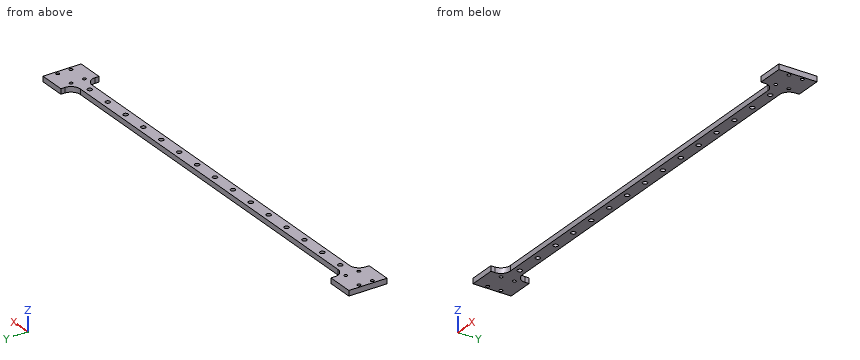
from build123d import *

# Parameters (mm, degrees)
SKETCH1_R           = 1.25
BOSS_EXTRUDE1_DEPTH = 4
FILLET1_R           = 7


with BuildPart() as part:
    # Sketch1 → Boss-Extrude1 (new body)
    with BuildSketch(Plane.XY):
        Polygon((-10, 14.45), (8.795857864, 14.45), (10, 14.45), (10, 4.5), (312, 4.5), (312, 14.45), (312.21, 14.45), (330.795857864, 14.45), (332, 14.45), (332, -14.45), (331.79, -14.45), (313.204142136, -14.45), (312, -14.45), (312, -4.5), (10, -4.5), (10, -14.45), (9.79, -14.45), (-8.795857864, -14.45), (-10, -14.45), (-10, -9.45), (-10, 9.45), align=None)
        with Locations((329.5, -5)):
            Circle(SKETCH1_R, mode=Mode.SUBTRACT)
        with Locations((314.5, 5)):
            Circle(SKETCH1_R, mode=Mode.SUBTRACT)
        with Locations((314.5, -5)):
            Circle(SKETCH1_R, mode=Mode.SUBTRACT)
        with Locations((329.5, 5)):
            Circle(SKETCH1_R, mode=Mode.SUBTRACT)
        with Locations((-7.5, -5)):
            Circle(SKETCH1_R, mode=Mode.SUBTRACT)
        with Locations((-7.5, 5)):
            Circle(SKETCH1_R, mode=Mode.SUBTRACT)
        with Locations((7.5, -5)):
            Circle(SKETCH1_R, mode=Mode.SUBTRACT)
        with Locations((7.5, 5)):
            Circle(SKETCH1_R, mode=Mode.SUBTRACT)
        with BuildLine():
            ThreePointArc((22.05, -1.4), (21, 1.75), (19.95, -1.4))
            ThreePointArc((19.95, -1.4), (21, -1.75), (22.05, -1.4))
        make_face(mode=Mode.SUBTRACT)
        with BuildLine():
            ThreePointArc((42.05, -1.4), (41, 1.75), (39.95, -1.4))
            ThreePointArc((39.95, -1.4), (41, -1.75), (42.05, -1.4))
        make_face(mode=Mode.SUBTRACT)
        with BuildLine():
            ThreePointArc((62.05, -1.4), (61, 1.75), (59.95, -1.4))
            ThreePointArc((59.95, -1.4), (61, -1.75), (62.05, -1.4))
        make_face(mode=Mode.SUBTRACT)
        with BuildLine():
            ThreePointArc((82.05, -1.4), (81, 1.75), (79.95, -1.4))
            ThreePointArc((79.95, -1.4), (81, -1.75), (82.05, -1.4))
        make_face(mode=Mode.SUBTRACT)
        with BuildLine():
            ThreePointArc((102.05, -1.4), (101, 1.75), (99.95, -1.4))
            ThreePointArc((99.95, -1.4), (101, -1.75), (102.05, -1.4))
        make_face(mode=Mode.SUBTRACT)
        with BuildLine():
            ThreePointArc((122.05, -1.4), (121, 1.75), (119.95, -1.4))
            ThreePointArc((119.95, -1.4), (121, -1.75), (122.05, -1.4))
        make_face(mode=Mode.SUBTRACT)
        with BuildLine():
            ThreePointArc((142.05, -1.4), (141, 1.75), (139.95, -1.4))
            ThreePointArc((139.95, -1.4), (141, -1.75), (142.05, -1.4))
        make_face(mode=Mode.SUBTRACT)
        with BuildLine():
            ThreePointArc((162.05, -1.4), (161, 1.75), (159.95, -1.4))
            ThreePointArc((159.95, -1.4), (161, -1.75), (162.05, -1.4))
        make_face(mode=Mode.SUBTRACT)
        with BuildLine():
            ThreePointArc((182.05, -1.4), (181, 1.75), (179.95, -1.4))
            ThreePointArc((179.95, -1.4), (181, -1.75), (182.05, -1.4))
        make_face(mode=Mode.SUBTRACT)
        with BuildLine():
            ThreePointArc((202.05, -1.4), (201, 1.75), (199.95, -1.4))
            ThreePointArc((199.95, -1.4), (201, -1.75), (202.05, -1.4))
        make_face(mode=Mode.SUBTRACT)
        with BuildLine():
            ThreePointArc((222.05, -1.4), (221, 1.75), (219.95, -1.4))
            ThreePointArc((219.95, -1.4), (221, -1.75), (222.05, -1.4))
        make_face(mode=Mode.SUBTRACT)
        with BuildLine():
            ThreePointArc((242.05, -1.4), (241, 1.75), (239.95, -1.4))
            ThreePointArc((239.95, -1.4), (241, -1.75), (242.05, -1.4))
        make_face(mode=Mode.SUBTRACT)
        with BuildLine():
            ThreePointArc((262.05, -1.4), (261, 1.75), (259.95, -1.4))
            ThreePointArc((259.95, -1.4), (261, -1.75), (262.05, -1.4))
        make_face(mode=Mode.SUBTRACT)
        with BuildLine():
            ThreePointArc((282.05, -1.4), (281, 1.75), (279.95, -1.4))
            ThreePointArc((279.95, -1.4), (281, -1.75), (282.05, -1.4))
        make_face(mode=Mode.SUBTRACT)
        with BuildLine():
            ThreePointArc((302.05, -1.4), (301, 1.75), (299.95, -1.4))
            ThreePointArc((299.95, -1.4), (301, -1.75), (302.05, -1.4))
        make_face(mode=Mode.SUBTRACT)
    extrude(amount=BOSS_EXTRUDE1_DEPTH)

    # Fillet1
    fillet1_edges = [part.edges().sort_by_distance(p)[0] for p in [
        (10, 4.5, 2),
        (312, 4.5, 2),
        (312, -4.5, 2),
        (10, -4.5, 2),
    ]]
    fillet(fillet1_edges, radius=FILLET1_R)


solid = part.part
The listing builds one solid part. Answer for the finished solid, in the listing's coordinates (mm). Round coordinates to 2 decimals unless told otherwise and drop trailing zeros. Order: outer loops, then holes, each group sorted by start corner. A loop starts at its lowest first (then second) coordinate and runs counter-clockwise, first axis right, second up. Notation, with made-up numbers: (-10.75, -34.75) -> (7.25, -34.75) arc R11 ccw to (7.25, -19.75) -> close; hole circle Ø4 at (45.5, -23.5). An arc over 180 degrees is marked (long way). One line per item, written item: value.
Item 1: Given P1, Ø2, axis at x = 7.5, y = -5, coming from the -Z side; P2, Ø1.5, axis at x = 118, z = 1.5, coming from the +Y side, each flat-ended and moving along its own axis, determine where each tip first touches the part or whether it passes through.
Taken from the geometry:
P1: passes through
P2: stops at y = 4.5
Item 2: Find section A-A, the plane x = 152. Give the vertices of the cut face in (y, z), then the cut area to 3 significant figures.
Taken from the geometry:
outline: (-4.5, 0) -> (4.5, 0) -> (4.5, 4) -> (-4.5, 4) -> close
area: 36.0 mm2
Item 3: Straight lines are drawn through the part: L1, parallel to X at y = 6, z = 0.9; L2, parallel to Y at x = 41, z = 2.55; L3, parallel to X at y = -5.25, z = 1. For each, find the intervals that lie inside material, in ascending order.
Taken from the geometry:
L1: x = -10 to -8.25, -6.75 to 6.75, 8.25 to 12.67, 309.33 to 313.75, 315.25 to 328.75, 330.25 to 332
L2: y = -4.5 to -1.75, 1.75 to 4.5
L3: x = -10 to -8.72, -6.28 to 6.28, 8.72 to 13.85, 308.15 to 313.28, 315.72 to 328.28, 330.72 to 332
Item 4: Find section B-B, the plane z = 2.15. State how many separate pieces and enclosed holes the cut face has, then the cut area to 3 significant figures.
Taken from the geometry:
separate pieces: 1
enclosed holes: 23
area: 3,730 mm2
